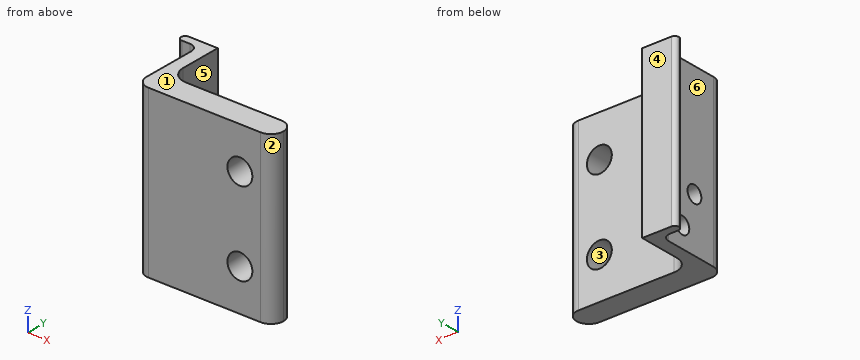
Autodesk Inventor part; units mm, degrees
ref_plane "YZ Plane" through (0, 0, 0) normal (1, 0, 0) x (0, 1, 0)
ref_plane "XZ Plane" through (0, 0, 0) normal (0, 1, 0) x (-1, 0, 0)
ref_plane "XY Plane" through (0, 0, 0) normal (0, 0, 1) x (1, 0, 0)
sketch "Sketch1" plane through (0, 0, 0) normal (0, 1, 0) x (-1, 0, 0)
  line L0 (0, 0) -> (33, 0)
  line L1 (33, 0) -> (33, -40)
  line L2 (33, -40) -> (0, -40)
  line L3 (0, -40) -> (0, 0)
  dimension "d0" = 33
  dimension "d1" = 40
extrude "Extrusion1" add sketch "Sketch1" along normal blind 6
sketch "Sketch2" plane through (0, 6, 0) normal (0, 1, 0) x (1, 0, 0)
  line L0 (-33, 0) -> (0, 0)
  line L1 (0, 40) -> (-33, 40)
  line L2 (-33, 0) -> (-30, 0)
  line L3 (-30, 0) -> (-30, 40)
  line L4 (-30, 40) -> (-33, 40)
  line L5 (-33, 40) -> (-33, 0)
  dimension "d4" = 3
extrude "Extrusion2" add sketch "Sketch2" along normal blind 14
sketch "Sketch3" plane through (-33, 0, -40) normal (-1, 0, 0) x (0, 0, 1)
  line L0 (0, 20) -> (40, 20)
  line L1 (40, 20) -> (0, 20)
  line L2 (0, 20) -> (0, 18)
  line L3 (0, 18) -> (40, 18)
  line L4 (40, 18) -> (40, 20)
  point P0 (40, 0)
  point P1 (0, 20)
  dimension "d7" = 40
  dimension "d8" = 2
extrude "Extrusion3" add sketch "Sketch3" along normal blind 5
fillet "Fillet1" radius 1 2 edges at (-38, 20, -20) (-38, 18, -20)
fillet "Fillet2" radius 4 1 edges at (-30, 6, -20)
fillet "Fillet3" radius 3 2 edges at (0, 6, -20) (0, 0, -20)
fillet "Fillet4" radius 3 1 edges at (-33, 0, -20)
sketch "Sketch4" plane through (0, 6, 0) normal (0, 1, 0) x (1, 0, 0)
  line L0 (-8, 0) -> (-8, 10)
  line L1 (-3, 40) -> (-30, 40)
  circle A0 centre (-8, 10) radius 3
  line L2 (-8, 40) -> (-8, 30)
  line L3 (-8, 40) -> (2, 40) construction
  circle A1 centre (-8, 30) radius 3
  point P0 (0, 0)
  dimension "d15" = 10
  dimension "d16" = 6
  dimension "d17" = 10
  dimension "d18" = 90
  dimension "d19" = 5
  dimension "d20" = 6
  dimension "d23" = 5
extrude "Extrusion4" cut sketch "Sketch4" against normal through all
fillet "Fillet5" radius 2 1 edges at (-33, 18, -20)
sketch "Sketch5" plane through (-33, 3, -40) normal (-1, 0, 0) x (0, 0, 1)
  line L0 (0, 5.5) -> (5, 5.5)
  line L1 (5, 5.5) -> (5, 9)
  line L2 (5, 5.5) -> (8.5, 5.5) construction
  line L3 (5, 5.5) -> (13, 5.5)
  circle A0 centre (5, 9) radius 2
  circle A1 centre (13, 5.5) radius 2
  line L4 (40, 0) -> (0, 0)
  line L5 (0, 7) -> (0, 17)
  line L6 (0, -3) -> (40, -3)
  dimension "d25" = 5
  dimension "d28" = 3.5
  dimension "d29" = 90
  dimension "d30" = 8
  dimension "d32" = 4
  dimension "d33" = 4
  dimension "d38" = 8.5
extrude "Extrusion5" cut sketch "Sketch5" against normal through all both and the other way through all
properties part number "Cable_Guide_Support"
CAD build for the part. Positions are in the model's coordinates, mm. Face numbers are marked on the shaded views. A direction names the side the tool comes from. Round coordinates to 2 decimals unless told otherwise and drop trailing zeros. Write each loop counter-clockwise with the first axis right and the second up, starting at its lowest first coordinate (ties: lowest second). Pieces come first, ordered by that corner, then holes.
(1) Slice it at B-B, the plane x = -8. Write the cut outline in (y, z), and give its area (3 significant figures).
(2) Mould opens along X. For the marked faces 1, 2 and 3 say: pulls with the +X half, pulls with the -X half, needs draft (parallel to the pull), parting line crosses it, or undercut.
(3) Drop flat-ended pins along their axis: P1, Ø1, axis at x = -25.5, z = -8, coming from the +Y side; P2, Ø5.5, axis at x = -8, z = -30, coming from the -Y side; P3, Ø8, axis at y = 12.5, z = -35, coming from the +X side; P4, Ø5, axis at y = 12, z = -35, coming from the +X side. Give the stop position or say it passes through.
(4) Probe line 1 along Z through (x, y) = (-8, 4.7); line 2 along Z through (x, y) = (-31.5, 8.5); line 3 along Z through (x, y) = (-32, 12). List the from-to ranges inside material, lowest first.
(5) 3-axis set-ups, long thin cutter, end or side, ignore diameter. For the marked faces 4, 5 and 6: which of +Z, -Z, +X, -X, +Y, -Y reach the whole face in a straight line?
(6) Slice it at D-D, the plane y = 4. Write the cut outline in (x, z).
From the geometry:
1. outline: (0, -40) - (6, -40) - (6, -33) - (0, -33) - close; (0, -27) - (6, -27) - (6, -13) - (0, -13) - close; (0, -7) - (6, -7) - (6, 0) - (0, 0) - close
1. area: 168 mm2
2. face 1: needs draft
2. face 2: pulls with the +X half
2. face 3: undercut
3. P1: stops at y = 6
3. P2: passes through
3. P3: stops at x = -29.71
3. P4: stops at x = -29.97
4. line 1: z = -40 to -33, -27 to -13, -7 to 0
4. line 2: z = -40 to -29, -25 to 0
4. line 3: z = -40 to -37, -33 to 0
5. face 4: +Z, -Z, +X, -X, +Y
5. face 5: +Z, -Z, +X, +Y
5. face 6: +Z, -Z, -X, -Y
6. outline: (-33, -40) - (-0.17, -40) - (-0.17, 0) - (-33, 0) - close; hole circle Ø6 at (-8, -30); hole circle Ø6 at (-8, -10)
